Autodesk Inventor part; units mm, degrees
ref_plane "Right_Connecting_Web_StartPlane" through (0, 0, 4) normal (0, 0, 1) x (1, 0, 0)
ref_plane "Right_Rod_Contact_Flange_StartPlane" through (0, 0, 10.5) normal (0, 0, 1) x (1, 0, 0)
ref_plane "Work Plane3" through (0, 0, 4) normal (0, 0, 1) x (1, 0, 0)
ref_plane "Right_Connecting_Web_StartPlane" through (0, 0, 4) normal (0, 0, 1) x (1, 0, 0)
sketch "Right_Connecting_Web_Profile" plane through (0, 0, 4) normal (0, 0, 1) x (1, 0, 0)
  line L0 (39, 0) -> (45, 0)
  line L1 (45, 0) -> (45, 80)
  line L2 (45, 80) -> (39, 80)
  line L3 (39, 80) -> (39, 0)
  point P0 (0, 0)
  dimension "d1" = 39
  dimension "d2" = 6
  dimension "d3" = 80
extrude "Right_Connecting_Web" add sketch "Right_Connecting_Web_Profile" along normal blind 8.5
ref_plane "Right_Rod_Contact_Flange_StartPlane" through (0, 0, 10.5) normal (0, 0, 1) x (1, 0, 0)
sketch "Right_Rod_Contact_Flange_Profile" plane through (0, 0, 10.5) normal (0, 0, 1) x (1, 0, 0)
  line L0 (39, 0) -> (51, 0)
  line L1 (51, 0) -> (51, 80)
  line L2 (51, 80) -> (39, 80)
  line L3 (39, 80) -> (39, 0)
  point P0 (0, 0)
  dimension "d7" = 39
  dimension "d8" = 12
  dimension "d9" = 80
extrude "Right_Rod_Contact_Flange" add sketch "Right_Rod_Contact_Flange_Profile" along normal blind 2
sketch "Original_Rod_Clearance_4x_Locations" plane through (0, 0, 0) normal (0, 0, 1) x (1, 0, 0)
  circle A0 centre (48, 5) radius 1.7
  circle A1 centre (48, 25) radius 1.7
  circle A2 centre (48, 45) radius 1.7
  circle A3 centre (48, 65) radius 1.7
  point P0 (0, 0)
  dimension "d12" = 48
  dimension "d13" = 5
  dimension "d14" = 3.4
  dimension "d15" = 48
  dimension "d16" = 25
  dimension "d17" = 3.4
  dimension "d18" = 48
  dimension "d19" = 45
  dimension "d20" = 3.4
  dimension "d21" = 48
  dimension "d22" = 65
  dimension "d23" = 3.4
extrude "Original_Rod_Clearance_4x" cut sketch "Original_Rod_Clearance_4x_Locations" along normal through all
ref_plane "Work Plane3" through (0, 0, 4) normal (0, 0, 1) x (1, 0, 0)
sketch "Deck_Assembly_M3_Locations" plane through (0, 0, 4) normal (0, 0, 1) x (1, 0, 0)
  circle A0 centre (41.5, 10) radius 1.25
  circle A1 centre (41.5, 30) radius 1.25
  circle A2 centre (41.5, 50) radius 1.25
  circle A3 centre (41.5, 70) radius 1.25
  point P0 (0, 0)
  dimension "d27" = 41.5
  dimension "d28" = 10
  dimension "d29" = 2.5
  dimension "d30" = 41.5
  dimension "d31" = 30
  dimension "d32" = 2.5
  dimension "d33" = 41.5
  dimension "d34" = 50
  dimension "d35" = 2.5
  dimension "d36" = 41.5
  dimension "d37" = 70
  dimension "d38" = 2.5
extrude "Four_Blind_M3_Tap_Bores" cut sketch "Deck_Assembly_M3_Locations" along normal blind 6.5
thread "Deck_M3x0_5_6H_1"
thread "Deck_M3x0_5_6H_2"
thread "Deck_M3x0_5_6H_3"
thread "Deck_M3x0_5_6H_4"
chamfer "Outer_End_2mm_45deg" distance 2 angle 45 1 edges at (51, 40, 10.5)
equation "\"d2\" = WebThickness"
equation "\"d3\" = ContactLength"
equation "\"d4\" = DropHeight"
equation "\"d8\" = RodWidth + WebThickness"
equation "\"d9\" = ContactLength"
equation "\"d10\" = RodFlangeThickness"
equation "\"d14\" = RodClearanceDiameter"
equation "\"d17\" = RodClearanceDiameter"
equation "\"d20\" = RodClearanceDiameter"
equation "\"d23\" = RodClearanceDiameter"
equation "\"d29\" = TapDrillDiameter"
equation "\"d32\" = TapDrillDiameter"
equation "\"d35\" = TapDrillDiameter"
equation "\"d38\" = TapDrillDiameter"
equation "\"d39\" = JoinThreadDepth"
equation "\"d41\" = JoinThreadDepth"
equation "\"d43\" = JoinThreadDepth"
equation "\"d45\" = JoinThreadDepth"
equation "\"d47\" = JoinThreadDepth"
equation "\"d49\" = OuterEndChamfer"
equation "\"d50\" = OuterEndChamfer"
equation "\"OverallWidth\" = 51"
equation "\"RodWidth\" = 6"
equation "\"ContactLength\" = 80"
equation "\"BaseThickness\" = 4"
equation "\"DropHeight\" = 8.5"
equation "\"WebThickness\" = 6"
equation "\"FingerStartX\" = 19.93338"
equation "\"FingerWidth\" = 13.5"
equation "\"FingerThickness\" = 6"
equation "\"FingerEndInset\" = 4"
equation "\"RodClearanceDiameter\" = 3.4"
equation "\"ClampFirstY\" = 41.82802"
equation "\"ClampPitch\" = 16"
equation "\"ClampHeight\" = BaseThickness + 0.5 * FingerThickness"
equation "\"TapDrillDiameter\" = 2.5"
equation "\"TapDepth\" = 6"
equation "\"RodHoleStart\" = 5"
equation "\"RodScrewPitch\" = 20"
equation "\"JoinLeftX\" = 9.5"
equation "\"JoinFirstY\" = 10"
equation "\"JoinPitch\" = 20"
equation "\"JoinThreadDepth\" = 6.5"
equation "\"JoinCountersinkDiameter\" = 6.2"
equation "\"d0\" = BaseThickness"
equation "\"d6\" = BaseThickness + DropHeight - RodFlangeThickness"
equation "\"d26\" = BaseThickness"
equation "\"RodFlangeThickness\" = 2"
equation "\"OuterEndChamfer\" = RodFlangeThickness"
properties part number "Right_Rod_Support"
Geometry: final body of the model. Coordinates: model frame, mm. A direction names the side the tool comes from. Round coordinates to 2 decimals unless told otherwise and drop trailing zeros. Write each loop counter-clockwise with the first axis right and the second up, starting at its lowest first coordinate (ties: lowest second). Pieces come first, ordered by that corner, then holes.
Item 1: Mould query, pull axis Y, two halves, no side actions, for faces 4 (the face through (45, 39, 7)), 5 (the face through (42, 80, 9)), 6 (the face through (41.34, 48.76, 7.2)). Classes: +Y half, -Y half, draft (parallel to the pull), parting line (faces both ways), or undercut.
Item 2: Section query C-C (x = 41.5). Return loops of the section in (y, z), plus the area to 3 significant figures.
Item 3: Material intervals for L1, parallel to Y at x = 41.5, z = 7.75; L2, parallel to Y at x = 48, z = 10.95; L3, parallel to X at y = 53, z = 6.75, sorted ascending.
Item 4: Pin query (flat end, axial travel): P1, Ø1.5, axis at y = 59, z = 10.5, coming from the +X side; P2, Ø0.8, axis at x = 41.5, y = 50, coming from the -Z side; P3, Ø2, axis at y = 45, z = 8, coming from the +X side. Return the tip coordinate at first contact, or that it passes through.
Item 5: Set-up query: faces 1 (the face through (47, 41, 10.5)), 2 (the face through (40.579, 29.155, 7.204)), 3 (the face through (42, 41, 4)). Return all of +Z, -Z, +X, -X, +Y, -Y with unobstructed straight access to the full face (end or side cutting, diameter ignored); none if empty.
Item 6: Section query A-A (y = 25). Return loops of the section in (x, z), plus the area to 3 significant figures.
Item 7: Section query B-B (z = 8). Return loops of the section in (x, y).
Completed:
1. face 4: draft
1. face 5: +Y half
1. face 6: undercut
2. outline: (0, 4) - (8.75, 4) - (8.75, 10.5) - (11.25, 10.5) - (11.25, 4) - (28.75, 4) - (28.75, 10.5) - (31.25, 10.5) - (31.25, 4) - (48.75, 4) - (48.75, 10.5) - (51.25, 10.5) - (51.25, 4) - (68.75, 4) - (68.75, 10.5) - (71.25, 10.5) - (71.25, 4) - (80, 4) - (80, 12.5) - (0, 12.5) - close
2. area: 615 mm2
3. L1: y = 0 to 8.75, 11.25 to 28.75, 31.25 to 48.75, 51.25 to 68.75, 71.25 to 80
3. L2: y = 0 to 3.3, 6.7 to 23.3, 26.7 to 43.3, 46.7 to 63.3, 66.7 to 80
3. L3: x = 39 to 45
4. P1: stops at x = 49.75
4. P2: stops at z = 10.5
4. P3: stops at x = 45
5. face 1: -Z, +X, +Y, -Y
5. face 2: -Z
5. face 3: -Z, +X, -X, +Y, -Y
6. outline: (39, 4) - (45, 4) - (45, 10.5) - (46.3, 10.5) - (46.3, 12.5) - (39, 12.5) - close; (49.7, 11.2) - (51, 12.5) - (49.7, 12.5) - close
6. area: 54.4 mm2
7. outline: (39, 0) - (45, 0) - (45, 80) - (39, 80) - close; hole circle Ø2.5 at (41.5, 10); hole circle Ø2.5 at (41.5, 30); hole circle Ø2.5 at (41.5, 50); hole circle Ø2.5 at (41.5, 70)
